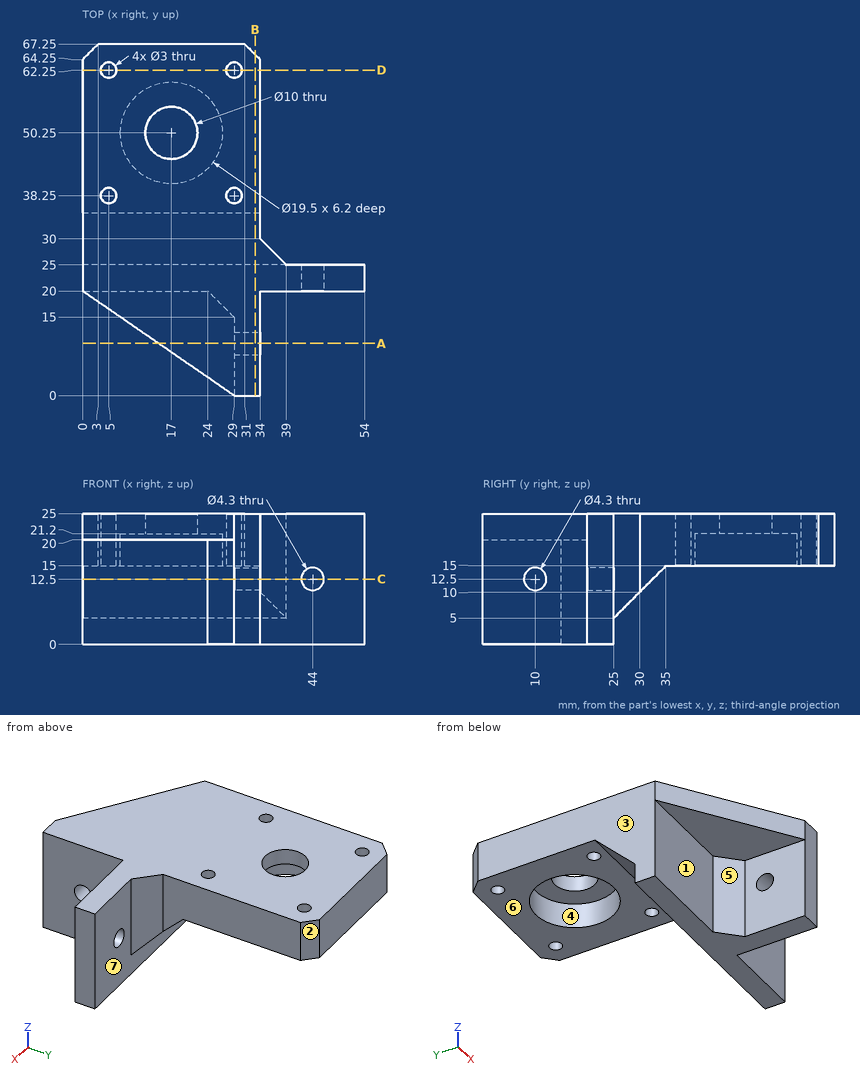
Answer from the drawing. Dimensions are ordinates in mm from the lowest x, y and z of the part. A direction names the side the tool comes from. Give positions to 0.01 mm unless a question says otherwise; leave off trailing zeros. Write each loop counter-clockwise with the first axis right and the second up, starting at its lowest first coordinate (ties: lowest second). Pieces come first, ordered by that corner, then holes.
1) Find the intervals of material crossed by L1, parallel to X at y = 62.25, z = 17.5; L2, parallel to Y at x = 29, z = 20.75; L3, parallel to X at y = 50.25, z = 22.7, in increasing order.
2) For a pull along X with two mould halves and no side action, classify the marked faces 1, 2, 3 and 4 as pulls with the +X half, pulls with the -X half, needs draft (parallel to the pull), parting line crosses it, or undercut.
3) Section B-B (x = 33) is taken. Write down the section's boundary in (y, z).
4) A tool of negligible diameter and unlimited length cuts with its end or side. For the marked faces 5, 6 and 7, from which of +Z, -Z, +X, -X, +Y, -Y can it reach the whole face along a straight path? Write none if from no direction.
5) Section D-D (y = 62.25) is taken. Write down the section's boundary in (x, z), and give its area (3 significant figures).
6) Section C-C (z = 12.5) is taken. Write down the section's boundary in (x, y), and give its area (3 significant figures).
7) Given P1, Ø5, axis at x = 29, y = 38.25, coming from the -Z side; P2, Ø12, axis at y = 41.5, z = 15.5, coming from the +X side; P3, Ø8, axis at x = 17, y = 50.25, coming from the -Z side; P4, Ø6, axis at x = 19, y = 13, coming from the -Z side, each flat-ended and moving along its own axis, determine where each tip first touches the part or whether it passes through.
8) Section A-A (y = 10) is taken. Write down the section's boundary in (x, z), and give its area (3 significant figures).
Response:
1. L1: x = 0 to 3.5, 6.5 to 27.5, 30.5 to 34
1. L2: y = 0 to 36.75, 39.75 to 60.75, 63.75 to 67.25
1. L3: x = 0 to 12, 22 to 34
2. face 1: needs draft
2. face 2: pulls with the +X half
2. face 3: pulls with the -X half
2. face 4: undercut
3. outline: (0, 0) - (25, 0) - (25, 5) - (35, 15) - (65.25, 15) - (65.25, 25) - (0, 25) - close; hole circle Ø4.3 at (10, 12.5)
4. face 5: -Z, -X, -Y
4. face 6: -Z, +X, -X, +Y
4. face 7: -Z, +X, +Y
5. outline: (0, 15) - (3.5, 15) - (3.5, 25) - (0, 25) - close; (6.5, 15) - (27.5, 15) - (27.5, 25) - (6.5, 25) - close; (30.5, 15) - (34, 15) - (34, 25) - (30.5, 25) - close
5. area: 280 mm2
6. outline: (0, 20) - (24, 20) - (29, 15) - (29, 12.15) - (34, 12.15) - (34, 20) - (41.85, 20) - (41.85, 25) - (39, 25) - (34, 30) - (34, 32.5) - (0, 32.5) - close; (29, 0) - (34, 0) - (34, 7.85) - (29, 7.85) - close; (46.15, 20) - (54, 20) - (54, 25) - (46.15, 25) - close
6. area: 607 mm2
7. P1: stops at z = 15
7. P2: stops at x = 34
7. P3: passes through
7. P4: stops at z = 20
8. outline: (14.5, 20) - (29, 20) - (29, 14.65) - (34, 14.65) - (34, 25) - (14.5, 25) - close; (29, 0) - (34, 0) - (34, 10.35) - (29, 10.35) - close
8. area: 176 mm2
